Here's the drawing with two shaded views (mm, measured from the low corner). I have some questions. A direction names the side the tool comes from. Coordinates: 2 decimals unless noted, no trailing zeros. Order: outer loops, then holes, each group sorted by start corner. A loop starts at its lowest first (then second) coordinate and runs counter-clockwise, first axis right, second up. Notation, with made-up numbers: (-17.5, -17) - (31.5, -17) arc R23 cw to (31.5, 16) - close; hole circle Ø10 at (-11, 64.25). An arc over 180 degrees is marked (long way). Answer as CSV lines item,"result". Start each with the question number.
1. I want a section at C-C, the plane z = 40. List the corners of the cut face in (x, y) for me.
2. Thinking about a two-plate mould opening in Y: for the marked faces 1, 2, 3 and 4, which applies, released by +Y, released by -Y, zero draft, split by the parting line, or undercut?
3. For pin 1 (4 mm diameter, centred on x = 28.5, y = 19.5, fed in from +Z); pin 2 (7 mm diameter, centred on x = 10, z = 40, fed in from -Y); pin 3 (10 mm diameter, centred on y = 20.5, z = 48.5, fed in from -X); pin 4 (6 mm diameter, centred on x = 69, y = 20.5, fed in from -Z), each with a flat end and sliding along its axis, tell me the tip position at first contact or that it passes through.
4. I want a section at D-D, the plane y = 6.5. Count the separate pieces of the cut face and the enclosed holes in it, and give its area (3 significant figures).
5. For the marked faces 5, 6 and 7, which set-ups out of +Z, -Z, +X, -X, +Y, -Y let a thin tool reach every point of the face, with its end or its side?
6. I need wall thicknesses on probe 1 along Z at (x, y) = (40, 8.5); probe 2 along Z at (x, y) = (10, 7.25); probe 3 along Y at (x, z) = (15.5, 42). Which ranges of each line are inside material? Lowest first, please.
7. I want a section at A-A, the plane z = 70. List the corners of the cut face in (x, y) for me, and give its area (3 significant figures).
8. I want a section at B-B, the plane x = 40. List the corners of the cut face in (y, z) for me.
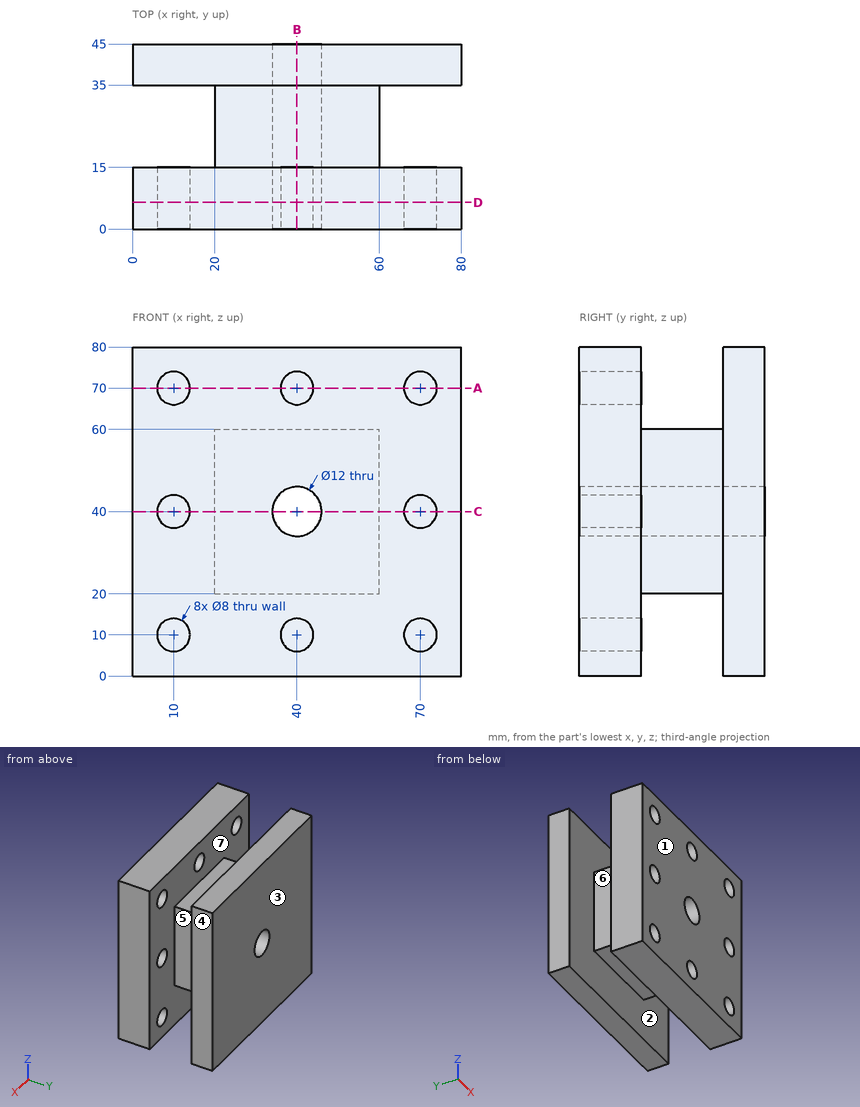
Solved:
1,outline,"(0, 0) - (6, 0) - (6, 15) - (0, 15) - close; (0, 35) - (20, 35) - (20, 15) - (14, 15) - (14, 0) - (34, 0) - (34, 45) - (0, 45) - close; (46, 0) - (66, 0) - (66, 15) - (60, 15) - (60, 35) - (80, 35) - (80, 45) - (46, 45) - close; (74, 0) - (80, 0) - (80, 15) - (74, 15) - close"
2,face 1,"released by -Y"
2,face 2,"undercut"
2,face 3,"released by +Y"
2,face 4,"zero draft"
3,pin 1,"stops at z = 60"
3,pin 2,"stops at y = 35"
3,pin 3,"stops at x = 20"
3,pin 4,"passes through"
4,separate pieces,"1"
4,enclosed holes,"9"
4,area,"5,880 mm2"
5,face 5,"+Z, -Z, +X"
5,face 6,"+Z, -Z, -X"
5,face 7,"none"
6,probe 1,"z = 0 to 6, 14 to 34, 46 to 66, 74 to 80"
6,probe 2,"z = 0 to 6, 14 to 36, 44 to 66, 74 to 80"
6,probe 3,"y = 0 to 15, 35 to 45"
7,outline,"(0, 0) - (6, 0) - (6, 15) - (0, 15) - close; (0, 35) - (80, 35) - (80, 45) - (0, 45) - close; (14, 0) - (36, 0) - (36, 15) - (14, 15) - close; (44, 0) - (66, 0) - (66, 15) - (44, 15) - close; (74, 0) - (80, 0) - (80, 15) - (74, 15) - close"
7,area,"1,640 mm2"
8,outline,"(0, 0) - (15, 0) - (15, 6) - (0, 6) - close; (0, 14) - (15, 14) - (15, 20) - (35, 20) - (35, 0) - (45, 0) - (45, 34) - (0, 34) - close; (0, 46) - (45, 46) - (45, 80) - (35, 80) - (35, 60) - (15, 60) - (15, 66) - (0, 66) - close; (0, 74) - (15, 74) - (15, 80) - (0, 80) - close"
